```python
from build123d import *

# Parameters (mm, degrees)
IZIM1_R                     = 46
IZIM1_R_2                   = 12
IZIM1_R_3                   = 10
Y_KSEKLIK_EKSTR_ZYON2_DEPTH = 83
Y_KSEKLIK_EKSTR_ZYON3_START = 2
IZIM1_4_R                   = 12
IZIM1_4_R_2                 = 10
Y_KSEKLIK_EKSTR_ZYON3_DEPTH = 2
Y_KSEKLIK_EKSTR_ZYON4_START = -83
IZIM1_7_R                   = 12
IZIM1_7_R_2                 = 10
Y_KSEKLIK_EKSTR_ZYON4_DEPTH = 2
IZIM2_R                     = 3
KES_EKSTR_ZYON1_DEPTH       = 100


with BuildPart() as part:
    # Çizim1 → Yükseklik-Ekstrüzyon2 (new body)
    # profile 1 of 2: a face of its own
    with BuildSketch(Plane.XY):
        Circle(IZIM1_R)
        Circle(IZIM1_R_2, mode=Mode.SUBTRACT)
    # profile 2 of 2: a face of its own
    with BuildSketch(Plane.XY):
        Circle(IZIM1_R_2)
        Circle(IZIM1_R_3, mode=Mode.SUBTRACT)
    extrude(amount=-Y_KSEKLIK_EKSTR_ZYON2_DEPTH)

    # Çizim1<4> → Yükseklik-Ekstrüzyon3 (add)
    with BuildSketch(Plane.XY.offset(Y_KSEKLIK_EKSTR_ZYON3_START)):
        Circle(IZIM1_4_R)
        Circle(IZIM1_4_R_2, mode=Mode.SUBTRACT)
    extrude(amount=-Y_KSEKLIK_EKSTR_ZYON3_DEPTH)

    # Çizim1<7> → Yükseklik-Ekstrüzyon4 (add)
    with BuildSketch(Plane.XY.offset(Y_KSEKLIK_EKSTR_ZYON4_START)):
        Circle(IZIM1_7_R)
        Circle(IZIM1_7_R_2, mode=Mode.SUBTRACT)
    extrude(amount=-Y_KSEKLIK_EKSTR_ZYON4_DEPTH)

    # Çizim2 → Kes-Ekstrüzyon1 (cut)
    with BuildSketch(Plane.XY):
        with Locations((-25.455844123, 25.455844123)):
            Circle(IZIM2_R)
        with Locations((25.455844123, 25.455844123)):
            Circle(IZIM2_R)
        with Locations((25.455844123, -25.455844123)):
            Circle(IZIM2_R)
        with Locations((-25.455844123, -25.455844123)):
            Circle(IZIM2_R)
    extrude(amount=-KES_EKSTR_ZYON1_DEPTH, mode=Mode.SUBTRACT)


solid = part.part
```
Input: part model. Units: mm. Frame: model coordinates. A direction names the side the tool comes from. Give positions to 0.01 mm unless a question says otherwise; leave off trailing zeros. Loops run counter-clockwise (first coordinate to the right, second up) from the corner with the lowest first, then second, coordinate; pieces in that order, holes last. Notation, with made-up numbers: M 25,12.25 L 54,12.25 A9 ccw 54,21.25 Z; hole C 23.25,-28 d7. An arc over 180 degrees is marked long. Answer as CSV lines item,"result". Start each with the question number.
1. Section D-D on z = -24. Return loops of the section in (x, y), plus the area to 3 significant figures.
2. Section B-B on x = 6.5. Return loops of the section in (y, z).
3. Reachability of faces 1 (the face through (10, -10, 0)), 2 (the face through (10, -10, -83)), 3 (the face through (28.23, -26.6, -40.92)) from +Z, -Z, +X, -X, +Y, -Y: full face, straight path, thin tool, end or side. Return the list, or none.
4. Section A-A on y = 0. Return loops of the section in (x, z).
5. Pull-direction query (Y, two-part tool) for faces 4 (the face through (28.23, 24.31, -40.92)), 5 (the face through (-5, 9, 2)), 6 (the face through (-11.99, 0.53, 1.01)); classes: released by +Y, released by -Y, zero draft, split by the parting line, or undercut.
6. Line query: L1, parallel to X at y = -27.5, z = -61.5; L2, parallel to Y at x = -26.5, z = -4; L3, parallel to X at y = -24.5, z = -67. Output: solid intervals per line, ascending.
7. Section C-C on y = -27. Return loops of the section in (x, z), plus the area to 3 significant figures.
8. Pin query (flat end, axial travel): P1, Ø3.5, axis at x = -25.46, y = -25.46, coming from the -Z side; P2, Ø9.5, axis at x = -25.46, y = 25.46, coming from the -Z side; P3, Ø1.5, axis at y = 3, z = -73, coming from the -X side; P4, Ø1, axis at x = -25, z = -49, coming from the -Y side. Return the tip coordinate at first contact, or that it passes through.
Computed values:
1,outline,"C 0,0 d92; hole C -25.46,-25.46 d6; hole C -25.46,25.46 d6; hole C 0,0 d20; hole C 25.46,-25.46 d6; hole C 25.46,25.46 d6"
1,area,"6,220 mm²"
2,outline,"M -45.54,-83 L -10.09,-83 L -10.09,-85 L -7.6,-85 L -7.6,2 L -10.09,2 L -10.09,0 L -45.54,0 Z; M 7.6,-85 L 10.09,-85 L 10.09,-83 L 45.54,-83 L 45.54,0 L 10.09,0 L 10.09,2 L 7.6,2 Z"
3,face 1,"+Z"
3,face 2,"-Z"
3,face 3,"+Z, -Z"
4,outline,"M -46,-83 L -12,-83 L -12,-85 L -10,-85 L -10,2 L -12,2 L -12,0 L -46,0 Z; M 10,-85 L 12,-85 L 12,-83 L 46,-83 L 46,0 L 12,0 L 12,2 L 10,2 Z"
5,face 4,"undercut"
5,face 5,"zero draft"
5,face 6,"split by the parting line"
6,L1,"x = -36.87 to -27.65, -23.26 to 23.26, 27.65 to 36.87"
6,L2,"y = -37.6 to -28.27, -22.64 to 22.64, 28.27 to 37.6"
6,L3,"x = -38.93 to -28.3, -22.61 to 22.61, 28.3 to 38.93"
7,outline,"M -37.24,-83 L -28.03,-83 L -28.03,0 L -37.24,0 Z; M -22.88,-83 L 22.88,-83 L 22.88,0 L -22.88,0 Z; M 28.03,-83 L 37.24,-83 L 37.24,0 L 28.03,0 Z"
7,area,"5,330 mm²"
8,P1,"passes through"
8,P2,"stops at z = -83"
8,P3,"stops at x = -45.94"
8,P4,"stops at y = -38.93"
